```python
from build123d import *

# Parameters (mm, degrees)
F0_R     = 4.5
F1_ANGLE = 180
F2_R     = 4.5
F3_DEPTH = 20
F4_R     = 4.5
F5_ANGLE = -180


with BuildPart() as f1:
    # F0 (on Top) → F1 (revolve)
    with BuildSketch(Plane.XY):
        Circle(F0_R)
    revolve(axis=Axis((15, -1.705776, 0), (0, -1, 0)), revolution_arc=F1_ANGLE)

    # F2 (on face) → F3 (join)
    with BuildSketch(Plane.XY):
        with Locations((29.965192, 0)):
            Circle(F2_R)
        Circle(F2_R)
    extrude(amount=F3_DEPTH)

    # F4 (on face) → F5 (revolve)
    with BuildSketch(Plane.XY.offset(20)):
        Circle(F4_R)
    revolve(axis=Axis((15, -0.568592, 20), (0, -1, 0)), revolution_arc=F5_ANGLE)


solid = f1.part
```
CAD build for the part. Positions are in the model's coordinates, mm. Round coordinates to 2 decimals unless told otherwise and drop trailing zeros. Order: outer loops, then holes, each group sorted by start corner. A loop starts at its lowest first (then second) coordinate and runs counter-clockwise, first axis right, second up. Notation, with made-up numbers: (55.25, 2) - (59.25, 2) arc R22 ccw to (59.25, 26) - close; hole circle Ø11 at (39, 86). An arc over 180 degrees is marked (long way). Answer as CSV lines item,"result". Start each with the question number.
1. Pin check, flat tips, straight feed: pin 1 (1.4 mm diameter, centred on x = 32, y = 2, fed in from +Z); pin 2 (5 mm diameter, centred on x = 27, y = -2, fed in from +Z); pin 3 (5 mm diameter, centred on y = 0.5, z = 25.5, fed in from +X); pin 4 (6 mm diameter, centred on x = 22.5, z = -11, fed in from -Y). Stop position of each tip, or through.
2. Pull direction Z, two halves, no side cores. Call faces 1 (the face through (25.47, 0.2, 9.86)), 2 (the face through (-0.59, 4.46, 9.86)): +Z half, -Z half, draft (parallel to the pull), parting line (faces both ways), or undercut.
3. Saw through at B-B, the plane z = 17. Write the cut outline in (x, y), and give its area (3 significant figures).
Model answer:
1,pin 1,"stops at z = 29.97"
1,pin 2,"stops at z = 36.78"
1,pin 3,"stops at x = 34.26"
1,pin 4,"stops at y = -4.5"
2,face 1,"undercut"
2,face 2,"undercut"
3,outline,"circle Ø9 at (0, 0); circle Ø9 at (29.97, 0)"
3,area,"127 mm²"
